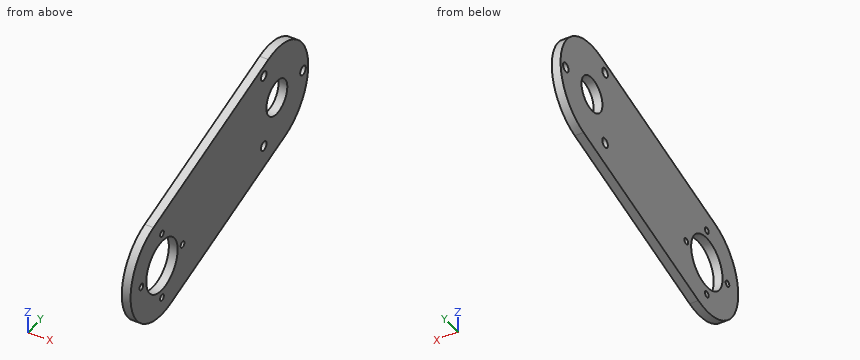
```python
from build123d import *

# Parameters (mm, degrees)
F0_R     = 19.05
F0_R_2   = 12.7
F1_DEPTH = 6.35
F2_D     = 4.4958
F3_D     = 6.7564


with BuildPart() as f1:
    # F0 (on Right) → F1 (new body)
    with BuildSketch(Plane.YZ):
        with BuildLine():
            Line((-129.2399760129, -75.5637942416), (10.2268421053, -36.7017942416))
            ThreePointArc((10.2268421053, -36.7017942416), (36.7017942416, 10.2268421053), (-10.2268421053, 36.7017942416))
            Line((-10.2268421053, 36.7017942416), (-149.6936602234, -2.1602057584))
            ThreePointArc((-149.6936602234, -2.1602057584), (-176.1686123598, -49.0888421053), (-129.2399760129, -75.5637942416))
        make_face()
        with Locations((-139.4668181181, -38.862)):
            Circle(F0_R, mode=Mode.SUBTRACT)
        Circle(F0_R_2, mode=Mode.SUBTRACT)
    extrude(amount=F1_DEPTH)

    # F2 (through all)
    with Locations(Plane(origin=(0, 0, 0), x_dir=(0, 1, 0), z_dir=(-1, 0, 0))):
        with Locations((-139.4668181181, 13.862), (-164.4668181181, 38.862), (-114.4668181181, 38.862), (-139.4668181181, 63.862)):
            Hole(F2_D / 2)

    # F3 (through all)
    with Locations(Plane(origin=(0, 0, 0), x_dir=(0, 1, 0), z_dir=(-1, 0, 0))):
        with Locations((-15.875, -27.4963065702), (-15.875, 27.4963065702), (31.75, 0)):
            Hole(F3_D / 2)


solid = f1.part
```
Design review of the part built by this model. Coordinates are the model's own, in mm. Round coordinates to 2 decimals unless told otherwise and drop trailing zeros. Order: outer loops, then holes, each group sorted by start corner. A loop starts at its lowest first (then second) coordinate and runs counter-clockwise, first axis right, second up. Notation, with made-up numbers: (15, -22.75) - (36, -22.75) arc R7 cw to (36, -9.75) - close; hole circle Ø4 at (53, 88). An arc over 180 degrees is marked (long way). Return JSON: item names as keys, results as strings.
Q1. Wall thickness on L1, parallel to Y at x = 1, z = -26.5; L2, parallel to Z at x = 1, y = 7; L3, parallel to Z at x = 5, y = -139: over which ranges is each line inside the solid? List them lowest first. Write a range as [from, to].
Computed values:
{"L1": "y = [-175.51, -153.96], [-124.97, -19.1], [-12.65, 27.37]", "L2": "z = [-37.6, -10.6], [10.6, 37.45]", "L3": "z = [-76.96, -66.06], [-61.66, -57.91], [-19.82, -16.06], [-11.66, 0.82]"}
Q2. For pin 1 Ø2 at (x, z) = (2.5, -45.5) entering from -Y; pin 2 Ø4 at (y, z) = (31.75, 0) entering from +X; pin 3 Ø1.5 at (x, y) = (4, -28) entering from +Z, all flat-tipped, find the tip position at first contact; note any pin that passes through.
Computed values:
{"pin 1": "stops at y = -177.15", "pin 2": "passes through", "pin 3": "stops at z = 31.96"}
Q3. Consider section A-A on y = 0. Write out the cut boundary in (x, z).
Computed values:
{"outline": "(0, -39.55) - (6.35, -39.55) - (6.35, -12.7) - (0, -12.7) - close; (0, 12.7) - (6.35, 12.7) - (6.35, 38.1) - (0, 38.1) - close"}
Q4. Consider section C-C on x = 1. Give the number of separate pieces and of enclosed holes in the cut face, plus the area to 3 significant figures.
Computed values:
{"separate pieces": "1", "enclosed holes": "9", "area": "13,800 mm2"}
Q5. Consider section D-D on y = -73. Write out the cut boundary in (x, z).
Computed values:
{"outline": "(0, -59.89) - (6.35, -59.89) - (6.35, 19.21) - (0, 19.21) - close"}
Q6. Consider section B-B on z = -47.5. Write out the cut boundary in (x, y).
Computed values:
{"outline": "(0, -176.57) - (6.35, -176.57) - (6.35, -156.45) - (0, -156.45) - close; (0, -122.49) - (6.35, -122.49) - (6.35, -28.53) - (0, -28.53) - close"}
